from build123d import *

# Parameters (mm, degrees)
SKETCH_1_W          = 166
SKETCH_1_H          = 138
EXTRUDE_1_DEPTH     = 3
SKETCH_2_W          = 166
SKETCH_2_H          = 138
SKETCH_2_W_2        = 159
SKETCH_2_H_2        = 131
EXTRUDE_2_DEPTH     = 55
CUT_EXTRUDE_4_REACH = 123.14
SKETCH_3_R          = 6.25
SKETCH_4_W          = 92
SKETCH_4_H          = 2.2
CUT_EXTRUDE_5_DEPTH = 1
SKETCH_5_W          = 92
SKETCH_5_H          = 2.2
CUT_EXTRUDE_6_DEPTH = 1
SKETCH_6_R          = 6.5
CUT_EXTRUDE_7_DEPTH = 10
SKETCH_7_R          = 5.5
CUT_EXTRUDE_8_DEPTH = 10
SKETCH_8_R          = 3.5
CUT_EXTRUDE_9_DEPTH = 10


with BuildPart() as part:
    # 스케치1 → 보스-돌출1 (new body)
    with BuildSketch(Plane.XY):
        Rectangle(SKETCH_1_W, SKETCH_1_H)
    extrude(amount=EXTRUDE_1_DEPTH)

    # 스케치2 → 보스-돌출2 (add)
    with BuildSketch(Plane.XY.offset(3)):
        Rectangle(SKETCH_2_W, SKETCH_2_H)
        Rectangle(SKETCH_2_W_2, SKETCH_2_H_2, mode=Mode.SUBTRACT)
    extrude(amount=EXTRUDE_2_DEPTH)

    # 스케치3 → 컷-돌출4 (cut, up to next)
    with BuildSketch(Plane.XY.offset(3), mode=Mode.PRIVATE) as cut_extrude_4_sk1:
        with Locations((-68, 54)):
            Circle(SKETCH_3_R)
    cut_extrude_4_tool1 = extrude(cut_extrude_4_sk1.sketch, amount=-CUT_EXTRUDE_4_REACH, mode=Mode.PRIVATE) & part.part
    # 스케치3 → 컷-돌출4 (cut, up to next)
    with BuildSketch(Plane.XY.offset(3), mode=Mode.PRIVATE) as cut_extrude_4_sk2:
        with Locations((-68, -54)):
            Circle(SKETCH_3_R)
    cut_extrude_4_tool2 = extrude(cut_extrude_4_sk2.sketch, amount=-CUT_EXTRUDE_4_REACH, mode=Mode.PRIVATE) & part.part
    # 스케치3 → 컷-돌출4 (cut, up to next)
    with BuildSketch(Plane.XY.offset(3), mode=Mode.PRIVATE) as cut_extrude_4_sk3:
        with Locations((68, -54)):
            Circle(SKETCH_3_R)
    cut_extrude_4_tool3 = extrude(cut_extrude_4_sk3.sketch, amount=-CUT_EXTRUDE_4_REACH, mode=Mode.PRIVATE) & part.part
    # 스케치3 → 컷-돌출4 (cut, up to next)
    with BuildSketch(Plane.XY.offset(3), mode=Mode.PRIVATE) as cut_extrude_4_sk4:
        with Locations((68, 54)):
            Circle(SKETCH_3_R)
    cut_extrude_4_tool4 = extrude(cut_extrude_4_sk4.sketch, amount=-CUT_EXTRUDE_4_REACH, mode=Mode.PRIVATE) & part.part
    add(cut_extrude_4_tool1.solids().sort_by_distance((-68, 54, 3))[0], mode=Mode.SUBTRACT)
    add(cut_extrude_4_tool2.solids().sort_by_distance((-68, -54, 3))[0], mode=Mode.SUBTRACT)
    add(cut_extrude_4_tool3.solids().sort_by_distance((68, -54, 3))[0], mode=Mode.SUBTRACT)
    add(cut_extrude_4_tool4.solids().sort_by_distance((68, 54, 3))[0], mode=Mode.SUBTRACT)

    # 스케치4 → 컷-돌출5 (cut)
    with BuildSketch(Plane.XZ.offset(-65.5)):
        with Locations((0, 55)):
            Rectangle(SKETCH_4_W, SKETCH_4_H)
    extrude(amount=-CUT_EXTRUDE_5_DEPTH, mode=Mode.SUBTRACT)

    # 스케치5 → 컷-돌출6 (cut)
    with BuildSketch(Plane(origin=(0, -65.5, 0), x_dir=(1, 0, 0), z_dir=(0, 1, 0))):
        with Locations((-0.014955436, -55)):
            Rectangle(SKETCH_5_W, SKETCH_5_H)
    extrude(amount=-CUT_EXTRUDE_6_DEPTH, mode=Mode.SUBTRACT)

    # 스케치6 → 컷-돌출7 (cut)
    with BuildSketch(Plane(origin=(0, 69, 0), x_dir=(1, 0, 0), z_dir=(0, 1, 0))):
        with Locations(Location((-25, -12, 0), (0, 0, 270))):
            Circle(SKETCH_6_R)
    extrude(amount=-CUT_EXTRUDE_7_DEPTH, mode=Mode.SUBTRACT)

    # 스케치7 → 컷-돌출8 (cut)
    with BuildSketch(Plane.ZY.offset(83)):
        with Locations((22, -24)):
            Circle(SKETCH_7_R)
    extrude(amount=-CUT_EXTRUDE_8_DEPTH, mode=Mode.SUBTRACT)

    # 스케치8 → 컷-돌출9 (cut)
    with BuildSketch(Plane(origin=(83, 0, 0), x_dir=(0, 0, -1), z_dir=(1, 0, 0))):
        with Locations((-22, -33)):
            Circle(SKETCH_8_R)
    extrude(amount=-CUT_EXTRUDE_9_DEPTH, mode=Mode.SUBTRACT)


solid = part.part
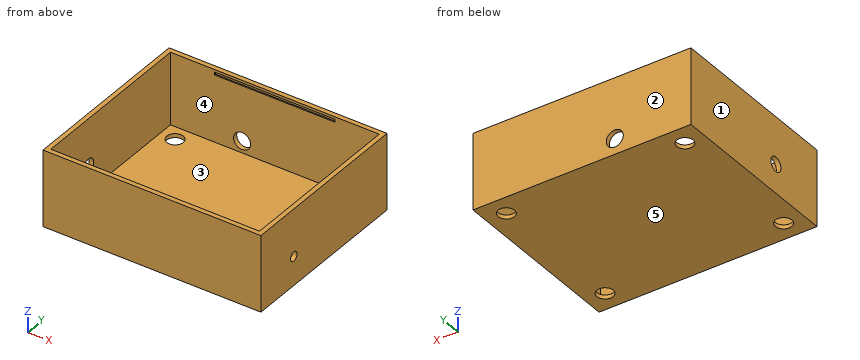
Here's how the part is built. I have some questions about the finished solid (model axes, mm). Face numbers are marked on the shaded views. A direction names the side the tool comes from. Coordinates: 2 decimals unless noted, no trailing zeros. Write each loop counter-clockwise with the first axis right and the second up, starting at its lowest first coordinate (ties: lowest second). Pieces come first, ordered by that corner, then holes.
1) If we section it at C-C (z = 48): List the corners of the cut face in (x, y) for me.
Filled in:
outline: (-83, -69) - (83, -69) - (83, 69) - (-83, 69) - close; hole (-79.5, -65.5) - (79.5, -65.5) - (79.5, 65.5) - (-79.5, 65.5) - close
2) Thinking about a two-plate mould opening in Y: for the marked faces 1, 2 and 3, which applies, +Y half, -Y half, draft (parallel to the pull), parting line (faces both ways), or undercut?
Filled in:
face 1: draft
face 2: +Y half
face 3: undercut
3) I'm going to push flat-ended pins straight in: pin 1 (6 mm diameter, centred on x = -33.5, y = 39, fed in from -Z); pin 2 (3 mm diameter, centred on x = 49, y = -28, fed in from +Z). Where does each tip first touch, or does it pass through?
Filled in:
pin 1: stops at z = 0
pin 2: stops at z = 3
4) If we section it at A-A (y = -33): List the corners of the cut face in (x, z) for me, plus the area to 4 significant figures.
Filled in:
outline: (-83, 0) - (83, 0) - (83, 18.5) - (79.5, 18.5) - (79.5, 3) - (-79.5, 3) - (-79.5, 58) - (-83, 58) - close; (79.5, 25.5) - (83, 25.5) - (83, 58) - (79.5, 58) - close
area: 858.5 mm2
5) If we section it at D-D (x = -68): List the corners of the cut face in (y, z) for me, plus the area to 3 significant figures.
Filled in:
outline: (-69, 0) - (-60.25, 0) - (-60.25, 3) - (-65.5, 3) - (-65.5, 58) - (-69, 58) - close; (-47.75, 0) - (47.75, 0) - (47.75, 3) - (-47.75, 3) - close; (60.25, 0) - (69, 0) - (69, 58) - (65.5, 58) - (65.5, 3) - (60.25, 3) - close
area: 724 mm2
6) Which directions (+Z, -Z, +X, -X, +Y, -Y) give clear straight access to the entire face, cutting with the end or side of a thin tool? Please do the marked faces 4 and 5.
Filled in:
face 4: +Z
face 5: -Z, +X, -X, +Y, -Y
7) If we section it at B-B (x = -25): List the corners of the cut face in (y, z) for me, plus the area to 3 significant figures.
Filled in:
outline: (-69, 0) - (69, 0) - (69, 5.5) - (65.5, 5.5) - (65.5, 3) - (-65.5, 3) - (-65.5, 53.9) - (-66.5, 53.9) - (-66.5, 56.1) - (-65.5, 56.1) - (-65.5, 58) - (-69, 58) - close; (65.5, 18.5) - (69, 18.5) - (69, 58) - (65.5, 58) - (65.5, 56.1) - (66.5, 56.1) - (66.5, 53.9) - (65.5, 53.9) - close
area: 749 mm2
8) If I drill on line 1 (Y direction, x = 68, z = 1.5); line 2 (Y direction, x = -3.5, z = 4); line 3 (X direction, y = 67.1, z = 12), over which ranges is the centre line in solid material (lowest first)?
Filled in:
line 1: y = -69 to -60.25, -47.75 to 47.75, 60.25 to 69
line 2: y = -69 to -65.5, 65.5 to 69
line 3: x = -83 to -31.5, -18.5 to 83
